```python
from build123d import *

# Parameters (mm, degrees)
SKETCH1_R             = 50.8
SKETCH1_R_2           = 6.35
BOSS_EXTRUDE1_DEPTH   = 10.16
BOSS_EXTRUDE1_2_DEPTH = 10.16
SKETCH2_W             = 25.4
SKETCH2_H             = 25.4
BOSS_EXTRUDE2_DEPTH   = 1524
SKETCH3_R             = 12.7
SKETCH8_R             = 12.7
SKETCH8_R_2           = 6.35
BOSS_EXTRUDE3_DEPTH   = 2.54


with BuildPart() as part:
    # Sketch1 → Boss-Extrude1 (new body)
    with BuildSketch(Plane(origin=(0, 0, 0), x_dir=(1, 0, 0), z_dir=(0, 1, 0))):
        with Locations((0, 317.5)):
            Circle(SKETCH1_R)
        with Locations((-38.1, 317.5)):
            Circle(SKETCH1_R_2, mode=Mode.SUBTRACT)
        with Locations((19.05, 350.495567884)):
            Circle(SKETCH1_R_2, mode=Mode.SUBTRACT)
        with Locations((19.05, 284.504432116)):
            Circle(SKETCH1_R_2, mode=Mode.SUBTRACT)
    extrude(amount=BOSS_EXTRUDE1_DEPTH)



with BuildPart() as body_2:
    # Sketch1 → Boss-Extrude1 2 (new body)
    with BuildSketch(Plane(origin=(0, 0, 0), x_dir=(1, 0, 0), z_dir=(0, 1, 0))):
        with Locations((0, -317.5)):
            Circle(SKETCH1_R)
        with Locations((19.05, -284.504432116)):
            Circle(SKETCH1_R_2, mode=Mode.SUBTRACT)
        with Locations((19.05, -350.495567884)):
            Circle(SKETCH1_R_2, mode=Mode.SUBTRACT)
        with Locations((-38.1, -317.5)):
            Circle(SKETCH1_R_2, mode=Mode.SUBTRACT)
    extrude(amount=BOSS_EXTRUDE1_2_DEPTH)


with BuildPart() as part_1:
    add(part.part)

    add(body_2.part)  # Boss-Extrude2 merges body 2
    # Sketch2 → Boss-Extrude2 (add)
    with BuildSketch(Plane(origin=(0, 10.16, 0), x_dir=(1, 0, 0), z_dir=(0, 1, 0))):
        with Locations((0, 317.5)):
            Rectangle(SKETCH2_W, SKETCH2_H)
        with Locations((0, -317.5)):
            Rectangle(SKETCH2_W, SKETCH2_H)
    extrude(amount=BOSS_EXTRUDE2_DEPTH)

    # Sweep1: sweep along a path in Sketch5
    with BuildLine(Plane(origin=(0, 0, 0), x_dir=(0, 0, -1), z_dir=(1, 0, 0))) as sweep1_path:
        Line((-304.8, 1407.16), (304.8, 1407.16))
    # Sketch3 → Sweep1 (sweep)
    with BuildSketch(Plane(origin=(0, 0, 304.8), x_dir=(-1, 0, 0), z_dir=(0, 0, -1))):
        with Locations((0, 1407.16)):
            Circle(SKETCH3_R)
    sweep(path=sweep1_path.line)

    # Sketch7 → Revolve2 (revolve)
    with BuildSketch(Plane(origin=(0, 0, 0), x_dir=(0, 0, -1), z_dir=(1, 0, 0))):
        with BuildLine():
            Line((-38.1, 1419.86), (-38.1, 1457.96))
            Line((-38.1, 1457.96), (-12.7, 1457.96))
            Line((-12.7, 1457.96), (-12.7, 1442.72))
            ThreePointArc((-12.7, 1442.72), (-9.724204897, 1435.535795103), (-2.54, 1432.56))
            Line((-2.54, 1432.56), (2.54, 1432.56))
            ThreePointArc((2.54, 1432.56), (9.724204897, 1435.535795103), (12.7, 1442.72))
            Line((12.7, 1442.72), (12.7, 1457.96))
            Line((12.7, 1457.96), (38.1, 1457.96))
            Line((38.1, 1457.96), (38.1, 1419.86))
            Line((38.1, 1419.86), (-38.1, 1419.86))
        make_face()
    revolve(axis=Axis((0, 1407.16, 304.8), (0, 0, -1)))

    # Sketch8 → Boss-Extrude3 (add)
    with BuildSketch(Plane(origin=(0, 10.16, 0), x_dir=(1, 0, 0), z_dir=(0, 1, 0))):
        with Locations((-38.1, -317.5)):
            Circle(SKETCH8_R)
        with Locations((-38.1, -317.5)):
            Circle(SKETCH8_R_2, mode=Mode.SUBTRACT)
        with Locations((19.05, -284.504432116)):
            Circle(SKETCH8_R)
        with Locations((19.05, -284.504432116)):
            Circle(SKETCH8_R_2, mode=Mode.SUBTRACT)
        with Locations((19.05, -350.495567884)):
            Circle(SKETCH8_R)
        with Locations((19.05, -350.495567884)):
            Circle(SKETCH8_R_2, mode=Mode.SUBTRACT)
        with Locations((19.05, 350.495567884)):
            Circle(SKETCH8_R)
        with Locations((19.05, 350.495567884)):
            Circle(SKETCH8_R_2, mode=Mode.SUBTRACT)
        with Locations((19.05, 284.504432116)):
            Circle(SKETCH8_R)
        with Locations((19.05, 284.504432116)):
            Circle(SKETCH8_R_2, mode=Mode.SUBTRACT)
        with Locations((-38.1, 317.5)):
            Circle(SKETCH8_R)
        with Locations((-38.1, 317.5)):
            Circle(SKETCH8_R_2, mode=Mode.SUBTRACT)
    extrude(amount=BOSS_EXTRUDE3_DEPTH)


solid = part_1.part
```
Source: CAD feature listing. Evaluate the final solid. Frame: model axes, mm. A direction names the side the tool comes from. Round coordinates to 2 decimals unless told otherwise and drop trailing zeros. Loops run counter-clockwise (first coordinate to the right, second up) from the corner with the lowest first, then second, coordinate; pieces in that order, holes last. Notation, with made-up numbers: M -5,88 L 9,88 A31 ccw 9,125 Z; hole C 66,-6 d6. An arc over 180 degrees is marked long. Use a Markdown table: item, result. Add a question column.
1. Line query: line 1 (Z direction, x = 19.05, y = 7); line 2 (Z direction, x = -38.1, y = 5); line 3 (Z direction, x = -12, y = 772). Output: solid intervals per line, ascending.
2. Contact query for flat-ended pins moving along their axis: P1, Ø20.5, axis at x = 20.5, z = -288, coming from the +Y side; P2, Ø20.5, axis at x = 6, y = 846, coming from the +Z side; P3, Ø5, axis at x = -10, z = 147.5, coming from the +Y side. Output: stop coordinate, or through.
3. Mould query, pull axis Y, two halves, no side actions, for faces 3 (the flat face through (-1, 0, -318)), 4 (the flat face through (22, 10.16, 317)), 5 (the flat face through (-11, 1397, 38.1)). Classes: pulls with the +Y half, pulls with the -Y half, needs draft (parallel to the pull), parting line crosses it, or undercut.
4. Section query B-B on z = 86.5. Return the cut outline in (x, y), then the cut area to 3 significant figures.
5. Section query A-A on y = 595. Return the cut outline in (x, z).
6. Reachability of faces 1 (the cylindrical face through (7.629, 1431.387, -0.036)), 2 (the flat face through (-1, 0, 317)) from +Z, -Z, +X, -X, +Y, -Y: full face, straight path, thin tool, end or side. Return the list, or none.
Reported:
| question | item | result |
|---|---|---|
| 1 | line 1 | z = -364.59 to -356.85, -344.15 to -290.85, -278.15 to -270.41, 270.41 to 278.15, 290.85 to 344.15, 356.85 to 364.59 |
| 1 | line 2 | z = -351.1 to -323.85, -311.15 to -283.9, 283.9 to 311.15, 323.85 to 351.1 |
| 1 | line 3 | z = -330.2 to -304.8, 304.8 to 330.2 |
| 2 | P1 | stops at y = 1414.66 |
| 2 | P2 | stops at z = 330.2 |
| 2 | P3 | stops at y = 1417.41 |
| 3 | face 3 | pulls with the -Y half |
| 3 | face 4 | undercut |
| 3 | face 5 | needs draft |
| 4 | outline | C 0,1407.16 d25.4 |
| 4 | area | 507 mm² |
| 5 | outline | M -12.7,-330.2 L 12.7,-330.2 L 12.7,-304.8 L -12.7,-304.8 Z; M -12.7,304.8 L 12.7,304.8 L 12.7,330.2 L -12.7,330.2 Z |
| 6 | face 1 | none |
| 6 | face 2 | +Z, -Z, +X, -X, -Y |
